CAD build for the part. Positions are in the model's coordinates, mm. Face numbers are marked on the shaded views. Round coordinates to 2 decimals unless told otherwise and drop trailing zeros. Write each loop counter-clockwise with the first axis right and the second up, starting at its lowest first coordinate (ties: lowest second). Pieces come first, ordered by that corner, then holes. Notation, with made-up numbers: (62, 40.5) - (97, 40.5) arc R21 ccw to (97, 62.5) - close; hole circle Ø10 at (5, 15). An arc over 180 degrees is marked (long way). Use one line per item in the form item = value. Start each with the question number.
Item 1: Band-saw the part on C-C, the plane x = 7. List the corners of the cut face in (y, z).
Item 2: Pull direction X, two halves, no side cores. Call the marked faces 1, 2 and 3: +X half, -X half, draft (parallel to the pull), parting line (faces both ways), or undercut.
Item 3: Band-saw the part on A-A, the plane y = -31.25. List the corners of the cut face in (x, z), and give its area (3 significant figures).
Item 4: Band-saw the part on B-B, the plane x = 0. List the corners of the cut face in (y, z), and give its area (4 significant figures).
Item 5: Drill centre lines: L1, parallel to Y at x = 15.5, z = 0.95; L2, parallel to Y at x = 0, z = 1.1; L3, parallel to X at y = 16, z = 3.75. Where is each one in solid material? Low to high.
Item 6: Pin check, flat tips, straight feed: pin 1 (0.8 mm diameter, centred on x = 24.5, z = 2, fed in from -Y); pin 2 (1 mm diameter, centred on x = 12, z = 3.5, fed in from -Y); pin 3 (1.4 mm diameter, centred on x = 27, y = 5.5, fed in from -Z). Stop position of each tip, or through.
from build123d import *

# Parameters (mm, degrees)
SKETCH_1_R          = 1.75
SKETCH_1_R_2        = 9.5
SKETCH_1_R_3        = 2.45
EXTRUDE_1_DEPTH     = 5
CHAMFER_1_SIZE      = 4
FILLET_1_R          = 3
CHAMFER_2_SIZE      = 1.7
CUT_EXTRUDE_1_DEPTH = 2


with BuildPart() as part:
    # Эскиз1 → Бобышка-Вытянуть1 (new body)
    with BuildSketch(Plane.XY):
        Polygon((-21.25, 21.25), (-21.25, -21.25), (-10, -21.25), (-10, -88.75), (10, -88.75), (10, -21.25), (21.25, -21.25), (21.25, -3), (28.75, -3), (28.75, 9.5), (21.25, 9.5), (21.25, 21.25), align=None)
        with Locations((-15.5, -15.5)):
            Circle(SKETCH_1_R, mode=Mode.SUBTRACT)
        with Locations((-15.5, 15.5)):
            Circle(SKETCH_1_R, mode=Mode.SUBTRACT)
        Circle(SKETCH_1_R_2, mode=Mode.SUBTRACT)
        with Locations((15.5, -15.5)):
            Circle(SKETCH_1_R, mode=Mode.SUBTRACT)
        with Locations((15.5, 15.5)):
            Circle(SKETCH_1_R, mode=Mode.SUBTRACT)
        with BuildLine():
            ThreePointArc((20.75, 0.75), (19.375, -0.625), (18, 0.75))
            Line((18, 0.75), (18, 5.75))
            ThreePointArc((18, 5.75), (19.375, 7.125), (20.75, 5.75))
            Line((20.75, 5.75), (20.75, 0.75))
        make_face(mode=Mode.SUBTRACT)
        with Locations((0, -31.25)):
            Circle(SKETCH_1_R_3, mode=Mode.SUBTRACT)
        with Locations((0, -81.25)):
            Circle(SKETCH_1_R_3, mode=Mode.SUBTRACT)
        with Locations((0, -61.25)):
            Circle(SKETCH_1_R_3, mode=Mode.SUBTRACT)
        with BuildLine():
            Line((24.5, 0.75), (24.5, 5.75))
            ThreePointArc((24.5, 5.75), (25.875, 7.125), (27.25, 5.75))
            Line((27.25, 5.75), (27.25, 0.75))
            ThreePointArc((27.25, 0.75), (25.875, -0.625), (24.5, 0.75))
        make_face(mode=Mode.SUBTRACT)
    extrude(amount=EXTRUDE_1_DEPTH)

    # Фаска1
    chamfer_1_edges = [part.edges().sort_by_distance(p)[0] for p in [
        (-21.25, -21.25, 2.5),
        (-21.25, 21.25, 2.5),
        (21.25, 21.25, 2.5),
        (21.25, -21.25, 2.5),
    ]]
    chamfer(chamfer_1_edges, length=CHAMFER_1_SIZE)

    # Скругление1
    fillet_1_edges = [part.edges().sort_by_distance(p)[0] for p in [
        (21.25, 9.5, 2.5),
        (28.75, 9.5, 2.5),
        (28.75, -3, 2.5),
        (21.25, -3, 2.5),
        (10, -21.25, 2.5),
        (-10, -21.25, 2.5),
    ]]
    fillet(fillet_1_edges, radius=FILLET_1_R)

    # Фаска2
    chamfer_2_edges = [part.edges().sort_by_distance(p)[0] for p in [
        (-17.25, -15.5, 5),
        (13.75, -15.5, 5),
        (13.75, 15.5, 5),
        (-17.25, 15.5, 5),
    ]]
    chamfer(chamfer_2_edges, length=CHAMFER_2_SIZE)

    # Эскиз2 → Вырез-Вытянуть1 (cut)
    with BuildSketch(Plane(origin=(0, 0, 0), x_dir=(-1, 0, 0), z_dir=(0, 0, -1))):
        with BuildLine():
            Line((-28.25, 5.75), (-28.25, 0.75))
            ThreePointArc((-28.25, 0.75), (-25.875, -1.625), (-23.5, 0.75))
            Line((-23.5, 0.75), (-23.5, 5.75))
            ThreePointArc((-23.5, 5.75), (-25.875, 8.125), (-28.25, 5.75))
        make_face()
        with BuildLine():
            Line((-17, 0.75), (-17, 5.75))
            ThreePointArc((-17, 5.75), (-19.375, 8.125), (-21.75, 5.75))
            Line((-21.75, 5.75), (-21.75, 0.75))
            ThreePointArc((-21.75, 0.75), (-19.375, -1.625), (-17, 0.75))
        make_face()
    extrude(amount=-CUT_EXTRUDE_1_DEPTH, mode=Mode.SUBTRACT)


solid = part.part
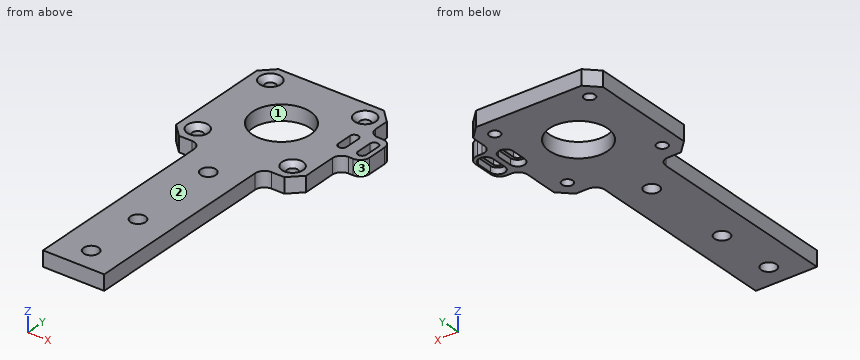
Determined:
q1.outline = (-88.75, 0) - (-6.42, 0) - (-6.42, 5) - (-88.75, 5) - close; (6.42, 0) - (21.25, 0) - (21.25, 5) - (6.42, 5) - close
q2.face_1 = undercut
q2.face_2 = draft
q2.face_3 = +X half
q3.outline = (-10, 0) - (-2.45, 0) - (-2.45, 5) - (-10, 5) - close; (2.45, 0) - (10, 0) - (10, 5) - (2.45, 5) - close
q3.area = 75.5 mm²
q4.outline = (-88.75, 0) - (-83.7, 0) - (-83.7, 5) - (-88.75, 5) - close; (-78.8, 0) - (-63.7, 0) - (-63.7, 5) - (-78.8, 5) - close; (-58.8, 0) - (-33.7, 0) - (-33.7, 5) - (-58.8, 5) - close; (-28.8, 0) - (-9.5, 0) - (-9.5, 5) - (-28.8, 5) - close; (9.5, 0) - (21.25, 0) - (21.25, 5) - (9.5, 5) - close
q4.area = 381.5 mm²
q5.L1 = -21.25 to -17.25, -13.75 to 13.75, 17.25 to 21.25
q5.L2 = -88.75 to -83.7, -78.8 to -63.7, -58.8 to -33.7, -28.8 to -9.5, 9.5 to 21.25
q5.L3 = -21.25 to -17.64, -13.36 to 13.36, 17.64 to 21.25
q6.pin_1 = -3
q6.pin_2 = -21.65
q6.pin_3 = 2
